Autodesk Inventor part; units mm, degrees
ref_plane "YZ Plane" through (0, 0, 0) normal (1, 0, 0) x (0, 1, 0)
ref_plane "XZ Plane" through (0, 0, 0) normal (0, 1, 0) x (-1, 0, 0)
ref_plane "XY Plane" through (0, 0, 0) normal (0, 0, 1) x (1, 0, 0)
sketch "草图1" plane through (0, 0, 0) normal (0, 0, 1) x (1, 0, 0)
  circle A0 centre (0, 0) radius 6
  dimension "d0" = 12
extrude "拉伸1" add sketch "草图1" along normal blind 1.5
sketch "草图2" plane through (0, 0, 1.5) normal (0, 0, 1) x (1, 0, 0)
  line L0 (0, -4.6188) -> (-4, -2.3094)
  line L1 (-4, -2.3094) -> (-4, 2.3094)
  line L2 (-4, 2.3094) -> (0, 4.6188)
  line L3 (0, 4.6188) -> (4, 2.3094)
  line L4 (4, 2.3094) -> (4, -2.3094)
  line L5 (4, -2.3094) -> (0, -4.6188)
  line L6 (0, 0) -> (0, 2.9591)
  dimension "d3" = 8
  dimension "d4" = 2.9591
extrude "拉伸2" add sketch "草图2" along normal blind 5
sketch "草图3" plane through (0, 0, 0) normal (0, 0, -1) x (-1, 0, 0)
  circle A0 centre (0, 0) radius 4
  dimension "d7" = 8
extrude "拉伸3" add sketch "草图3" along normal blind 25
thread "螺纹1"
chamfer "倒角1" distance 0.5 angle 45 1 edges at (4, 0, -25)
fillet "圆角1" radius 0.5 13 edges at (-6, 0, 1.5) (4, 0, 6.5) (2, 3.4641, 6.5) (-2, 3.4641, 6.5) (-4, 0, 6.5) (-2, -3.4641, 6.5) (2, -3.4641, 6.5) (4, 2.3094, 4) (0, 4.6188, 4) (4, -2.3094, 4) (0, -4.6188, 4) (-4, -2.3094, 4) (-4, 2.3094, 4)
properties part number "装填斗固定螺丝"
Here's how the part is built. I have some questions about the finished solid (model axes, mm). A direction names the side the tool comes from. Give positions to 0.01 mm unless a question says otherwise; leave off trailing zeros. Order: outer loops, then holes, each group sorted by start corner. A loop starts at its lowest first (then second) coordinate and runs counter-clockwise, first axis right, second up. Notation, with made-up numbers: (39.25, 44.5) -> (52.25, 44.5) arc R19 ccw to (52.25, 50.5) -> close; hole circle Ø8 at (60, -8.75). An arc over 180 degrees is marked (long way). Use CSV: the item, a comma, the result in double quotes. Start each with the question number.
Item 1: Suppose I cut it at A-A (z = 4). List the corners of the cut face in (x, y) for me.
Item 2: Suppose I cut it at B-B (y = 0). List the corners of the cut face in (x, z) for me, and give its area (3 significant figures).
Item 3: If I drill on probe 1 along X at (y, z) = (-1.25, 4); probe 2 along Z at (x, y) = (-1.5, -5); probe 3 along Y at (x, z) = (0.5, -13), over which ranges is the centre line in solid material (lowest first)? Write a range as [from, to].
Item 4: Suppose I cut it at C-C (z = -3.5). List the corners of the cut face in (x, y) for me, and give its area (3 significant figures).
Item 5: I'm going to push flat-ended pins straight in: P1, Ø4, axis at x = -2, y = 4, coming from the -Z side; P2, Ø1.5, axis at x = 1.5, z = 1.5, coming from the +Y side; P3, Ø1.2, axis at y = -1, z = 2.5, coming from the -X side; P4, Ø1.5, axis at x = -4.5, y = 3, coming from the +Z side. Where does each tip first touch, or does it pass through?
Item 6: On a 3-axis mill with a long thin cutter (end or side, diameter ignored), from which of +Z, -Z, +X, -X, +Y, -Y can I reach the whole of each face in a straight line? I mean faces 1 (the flat face through (-1.975, -3.478, 3.718)), 2 (the flat face through (-4, 0, 4)), 3 (the flat face through (-1.42, -3.92, 0)), 4 (the flat face through (1.975, 3.478, 3.718)). Say none if no direction works.
Answer block:
1,outline,"(-4, -2.02) arc R0.5 ccw to (-3.75, -2.45) -> (-0.25, -4.47) arc R0.5 ccw to (0.25, -4.47) -> (3.75, -2.45) arc R0.5 ccw to (4, -2.02) -> (4, 2.02) arc R0.5 ccw to (3.75, 2.45) -> (0.25, 4.47) arc R0.5 ccw to (-0.25, 4.47) -> (-3.75, 2.45) arc R0.5 ccw to (-4, 2.02) -> close"
2,outline,"(-6, 0) -> (-4, 0) -> (-4, -24.5) -> (-3.5, -25) -> (3.5, -25) -> (4, -24.5) -> (4, 0) -> (6, 0) -> (6, 1) arc R0.5 ccw to (5.5, 1.5) -> (4, 1.5) -> (4, 6) arc R0.5 ccw to (3.5, 6.5) -> (-3.5, 6.5) arc R0.5 ccw to (-4, 6) -> (-4, 1.5) -> (-5.5, 1.5) arc R0.5 ccw to (-6, 1) -> close"
2,area,"258 mm^2"
3,probe 1,"x = [-4, 4]"
3,probe 2,"z = [0, 1.5]"
3,probe 3,"y = [-3.97, 3.97]"
4,outline,"circle Ø8 at (0, 0)"
4,area,"50.3 mm^2"
5,P1,"stops at z = -25"
5,P2,"stops at y = 5.93"
5,P3,"stops at x = -4"
5,P4,"stops at z = 1.5"
6,face 1,"+Z, -X, -Y"
6,face 2,"+Z, -X, +Y, -Y"
6,face 3,"-Z"
6,face 4,"+Z, +X, +Y"
